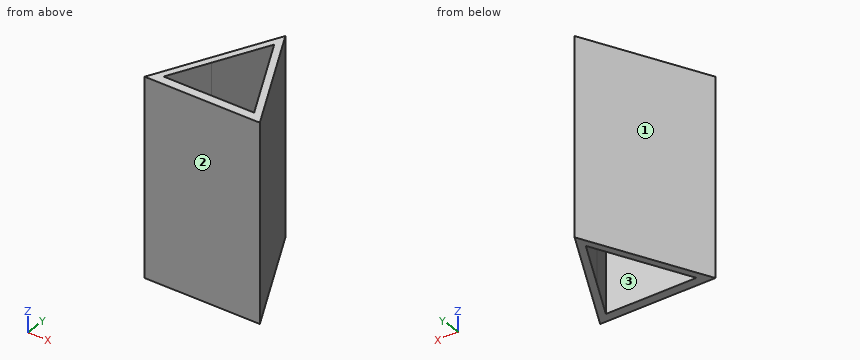
Autodesk Inventor part; units mm, degrees
ref_plane "YZ Plane" through (0, 0, 0) normal (1, 0, 0) x (0, 1, 0)
ref_plane "XZ Plane" through (0, 0, 0) normal (0, 1, 0) x (-1, 0, 0)
ref_plane "XY Plane" through (0, 0, 0) normal (0, 0, 1) x (1, 0, 0)
sketch "Boceto1" plane through (0, 0, 0) normal (0, 0, 1) x (1, 0, 0)
  line L0 (0, 0) -> (50, 0)
  line L1 (50, 0) -> (50, 50)
  line L2 (50, 50) -> (0, 50)
  line L3 (0, 50) -> (0, 0)
  line L4 (0, 0) -> (25, 50)
  line L5 (50, 0) -> (25, 50)
  dimension "d0" = 50
  dimension "d1" = 50
extrude "Extrusión1" add sketch "Boceto1" along normal blind 85 contours L4 L5 L0
sketch "Boceto2" plane through (0, 0, 85) normal (0, 0, 1) x (1, 0, 0)
  line L0 (25, 4) -> (47.7159, 4)
  line L1 (50, 0) -> (25, 50)
  line L2 (37.5, 25) -> (38.8416, 22.3167)
  line L3 (38.8416, 22.3167) -> (36.1584, 20.9751)
  line L4 (36.1584, 20.9751) -> (44.6459, 4)
  line L5 (25, 4) -> (2, 4)
  line L6 (25, 50) -> (0, 0)
  line L7 (11.1584, 22.3167) -> (13.8416, 20.9751)
  line L8 (13.8416, 20.9751) -> (5.3541, 4)
  line L9 (13.8416, 20.9751) -> (25, 43.2918)
  line L10 (25, 43.2918) -> (36.1584, 20.9751)
  dimension "d4" = 3
  dimension "d5" = 3
  dimension "d6" = 3
extrude "Extrusión2" cut sketch "Boceto2" against normal blind 85 contours L5 L8 L9 L10 L4 L0
properties part number "Aspax2"
The listing builds one solid part. Answer for the finished solid, in the listing's coordinates (mm). Face numbers are marked on the shaded views. Give positions to 0.01 mm unless a question says otherwise; leave off trailing zeros. Write each loop counter-clockwise with the first axis right and the second up, starting at its lowest first coordinate (ties: lowest second). Pieces come first, ordered by that corner, then holes. Notation, with made-up numbers: M -0.75,20 L 35.25,20 A21 ccw 35.25,30 Z; hole C 47,68.5 d4. An arc over 180 degrees is marked long. Write each question's results on one line, items separated by ' | '.
Q1. Flat-ended cylindrical pins translate along their axes: P1, Ø12, axis at y = 13.5, z = 18.5, coming from the +X side; P2, Ø1.5, axis at x = 12, z = 65, coming from the +Y side; P3, Ø8, axis at x = 9, z = 30.5, coming from the +Y side. Find the tip coordinate at first contact, or state that the pin passes through.
Output values:
P1: x = 46.25 | P2: y = 25.5 | P3: y = 26
Q2. Section A-A, the plane x = 26.5 is taken. Write down the section's boundary in (y, z).
Output values:
outline: M 0,0 L 4,0 L 4,85 L 0,85 Z; M 40.29,0 L 47,0 L 47,85 L 40.29,85 Z
Q3. Consider L1, parallel to X at y = 35, z = 73; L2, parallel to Y at x = 32, z = 9.5; L3, parallel to X at y = 32.5, z = 40. Determine where each line is inside the solid, lowest interval first. Write a range as from..to.
Output values:
L1: 17.5..20.85, 29.15..32.5 | L2: 0..4, 29.29..36 | L3: 16.25..19.6, 30.4..33.75
Q4. Section B-B, the plane y = 18.5 is taken. Write down the section's boundary in (x, z).
Output values:
outline: M 9.25,0 L 12.6,0 L 12.6,85 L 9.25,85 Z; M 37.4,0 L 40.75,0 L 40.75,85 L 37.4,85 Z
Q5. For a pull along X with two mould halves and no side action, classify the marked faces 1, 2 and 3 as released by +X, released by -X, zero draft, split by the parting line, or undercut.
Output values:
face 1: released by -X | face 2: zero draft | face 3: undercut
Q6. Section C-C, the plane z = 72 is taken. Write down the section's boundary in (x, y).
Output values:
outline: M 0,0 L 50,0 L 25,50 Z; hole M 5.35,4 L 44.65,4 L 36.16,20.98 L 25,43.29 L 13.84,20.98 Z
